from build123d import *

# Parameters (mm, degrees)
EXTRUDE_417_DEPTH = 15
SKETCH_2_R        = 20
EXTRUDE_1_DEPTH   = 90
EXTRUDE_2_DEPTH   = 15
SKETCH_6_R        = 20
EXTRUDE_5_DEPTH   = 72
EXTRUDE_6_DEPTH   = 10
FILLET_5_R        = 5


with BuildPart() as part:
    # Эскиз1 → Extrude 417 (new body)
    with BuildSketch(Plane(origin=(0, 0, 0), x_dir=(0, 0, -1), z_dir=(1, 0, 0))):
        Polygon((26.558112383, 0), (13.279056191, 23), (-13.279056191, 23), (-26.558112383, 0), (-13.279056191, -23), (13.279056191, -23), align=None)
    extrude(amount=EXTRUDE_417_DEPTH)

    # Эскиз2 → Бобышка-Вытянуть1 (add)
    with BuildSketch(Plane(origin=(15, 0, 0), x_dir=(0, 0, -1), z_dir=(1, 0, 0))):
        with Locations(Location((0, 0, 0), (0, 0, 180))):
            Circle(SKETCH_2_R)
    extrude(amount=EXTRUDE_1_DEPTH)

    # Эскиз3 → Бобышка-Вытянуть2 (add)
    with BuildSketch(Plane(origin=(105, 0, 0), x_dir=(0, 0, -1), z_dir=(1, 0, 0))):
        Polygon((26.558112383, 0), (13.279056191, 23), (-13.279056191, 23), (-26.558112383, 0), (-13.279056191, -23), (13.279056191, -23), align=None)
    extrude(amount=EXTRUDE_2_DEPTH)

    # Эскиз6 → Бобышка-Вытянуть5 (add)
    with BuildSketch(Plane(origin=(24.626459013, -31.520430144, 0), x_dir=(0, 0, 1), z_dir=(-0.6156614753256595, 0.7880107536067209, 0))):
        with Locations(Location((0, 40, 0), (0, 0, 270))):
            Circle(SKETCH_6_R)
    extrude(amount=-EXTRUDE_5_DEPTH)

    # Эскиз7 → Бобышка-Вытянуть6 (add)
    with BuildSketch(Plane(origin=(68.954085236, -88.257204404, 0), x_dir=(0, 0, -1), z_dir=(0.6156614753256596, -0.788010753606721, 0))):
        Polygon((6.635774784, 51.493499074), (-6.635774784, 51.493499074), (-13.271549568, 40), (-6.635774784, 28.506500926), (6.635774784, 28.506500926), (13.271549568, 40), align=None)
    extrude(amount=EXTRUDE_6_DEPTH)

    # Скругление5
    fillet_5_edges = [part.edges().sort_by_distance(p)[0] for p in [
        (116.234730453, -51.317515884, 0),
    ]]
    fillet(fillet_5_edges, radius=FILLET_5_R)


solid = part.part
Input: part model. Units: mm. Frame: model coordinates. A direction names the side the tool comes from. Give positions to 0.01 mm unless a question says otherwise; leave off trailing zeros. Order: outer loops, then holes, each group sorted by start corner. A loop starts at its lowest first (then second) coordinate and runs counter-clockwise, first axis right, second up. Notation, with made-up numbers: (-19, -13.75) - (1, -13.75) arc R30 ccw to (1, 23.25) - close; hole circle Ø4 at (72, 58). An arc over 180 degrees is marked (long way). Write each question's results on one line, items separated by ' | '.
Item 1: Section C-C (x = 9). Return loops of the section in (y, z), and give its area (3 significant figures).
A:
outline: (-23, -13.28) - (0, -26.56) - (23, -13.28) - (23, 13.28) - (0, 26.56) - (-23, 13.28) - close | area: 1,830 mm^2
Item 2: Section A-A (x = 39.5). Return loops of the section in (y, z), and give its area (3 significant figures).
A:
outline: circle Ø40 at (0, 0) | area: 1,260 mm^2
Item 3: Contact query for flat-ended pins moving along their axis: pin 1 Ø8 at (y, z) = (-57.5, -15.5) entering from +X; pin 2 Ø1 at (y, z) = (-41.5, -3) entering from +X; pin 3 Ø10 at (y, z) = (-39.5, -9) entering from -X. Output: stop coordinate, or through.
A:
pin 1: stops at x = 110.07 | pin 2: stops at x = 108.68 | pin 3: stops at x = 54.24
Item 4: Material intervals for line 1 along X through (y, z) = (6.5, -20.5); line 2 along Y through (x, z) = (86, -11.5); line 3 along Y through (x, z) = (96, -4), sorted ascending.
A:
line 1: x = 0 to 15, 105 to 120 | line 2: y = -70.96 to -18.53, -16.36 to 16.36 | line 3: y = -76.57 to -26.07, -19.6 to 19.6
Item 5: Draft query along X for faces 5 (the flat face through (99.04, -71, 10)), 6 (the flat face through (107.975, -64.027, -10)), 7 (the flat face through (50.15, -11.58, -16.88)), 8 (the flat face through (7, 23, 0)). Return one class per face: released by +X, released by -X, zero draft, split by the parting line, or undercut.
A:
face 5: undercut | face 6: released by +X | face 7: undercut | face 8: zero draft
Item 6: Section B-B (z = 0). Return loops of the section in (x, y), and give its area (3 significant figures).
A:
outline: (0, -23) - (15, -23) - (15, -20) - (41.01, -20) - (81.64, -72) arc R5 ccw to (88.65, -72.87) - (91.42, -70.71) - (97.57, -78.59) - (115.69, -64.43) - (109.53, -56.55) - (112.29, -54.4) arc R5 ccw to (113.16, -47.38) - (91.77, -20) - (105, -20) - (105, -23) - (120, -23) - (120, 23) - (105, 23) - (105, 20) - (15, 20) - (15, 23) - (0, 23) - close | area: 7,410 mm^2
Item 7: Access query for faces 1 (the flat face through (94.45, -74.59, 0.09)), 2 (the flat face through (98.9, -71.1, -9.9)), 3 (the flat face through (112, -23, 0)), 4 (the flat face through (7.4, -11.34, 20.01)). Directions: +Z, -Z, +X, -X, +Y, -Y. A direction counts if a zero-diameter tool reaches every point of the face in a straight line with its end or side. Return the directions, or none.
A:
face 1: +Z, -Z, -Y | face 2: -Z, -Y | face 3: +Z, -Z, +X | face 4: +Z, -X, -Y
